Autodesk Inventor part; units mm, degrees
ref_plane "YZ Plane" through (0, 0, 0) normal (1, 0, 0) x (0, 1, 0)
ref_plane "XZ Plane" through (0, 0, 0) normal (0, 1, 0) x (-1, 0, 0)
ref_plane "XY Plane" through (0, 0, 0) normal (0, 0, 1) x (1, 0, 0)
sketch "Sketch1" plane through (0, 0, 0) normal (0, 0, 1) x (1, 0, 0)
  circle A0 centre (45.5, -15.3826) radius 3
  circle A1 centre (-45.5, -15.3826) radius 3
  line L0 (44.6636, 0.7689) -> (35.6636, 0.7689)
  line L1 (33.6636, 2.7689) -> (33.6636, 5.2689)
  line L2 (46.6636, 5.2689) -> (46.6636, 2.7689)
  line L3 (29.9455, -2.1666) -> (-2.0545, -2.1666)
  line L4 (-4.0545, -0.1666) -> (-4.0545, 2.8334)
  line L5 (31.9455, 2.8334) -> (31.9455, -0.1666)
  circle A2 centre (89.024, -15.4039) radius 1.5
  circle A3 centre (65.024, -15.4039) radius 1.5
  circle A4 centre (89.024, 8.5961) radius 1.5
  circle A5 centre (65.024, 8.5961) radius 1.5
  arc A6 (67.8322, 7.6809) -> (67.8322, -14.4886) centre (77.024, -3.4039) ccw
  line L6 (69.3366, 7.4111) -> (71.8641, 3.0334)
  arc A7 (71.8641, 3.0334) -> (71.8641, -9.8411) centre (77.024, -3.4039) ccw
  line L7 (71.8641, -9.8411) -> (69.3366, -14.2188)
  arc A8 (67.8322, -14.4886) -> (69.3366, -14.2188) centre (68.4705, -13.7188) ccw
  arc A9 (69.3366, 7.4111) -> (67.8322, 7.6809) centre (68.4705, 6.9111) ccw
  arc A10 (91.2195, -0.986) -> (72.0202, 10.0988) centre (77.024, -3.4039) ccw
  arc A11 (72.0202, 10.0988) -> (71.5016, 8.6611) centre (72.3677, 9.1611) ccw
  line L8 (74.0291, 4.2834) -> (71.5016, 8.6611)
  arc A12 (85.1787, -2.1539) -> (74.0291, 4.2834) centre (77.024, -3.4039) ccw
  line L9 (90.2337, -2.1539) -> (85.1787, -2.1539)
  arc A13 (90.2337, -2.1539) -> (91.2195, -0.986) centre (90.2337, -1.1539) ccw
  line L10 (85.1787, -4.6539) -> (90.2337, -4.6539)
  arc A14 (91.2195, -5.8218) -> (90.2337, -4.6539) centre (90.2337, -5.6539) ccw
  arc A15 (72.0202, -16.9065) -> (91.2195, -5.8218) centre (77.024, -3.4039) ccw
  arc A16 (71.5016, -15.4688) -> (72.0202, -16.9065) centre (72.3677, -15.9688) ccw
  line L11 (71.5016, -15.4688) -> (74.0291, -11.0911)
  arc A17 (74.0291, -11.0911) -> (85.1787, -4.6539) centre (77.024, -3.4039) ccw
  circle A18 centre (-64.8953, -15.374) radius 1.5
  circle A19 centre (-88.8953, -15.374) radius 1.5
  circle A20 centre (-88.8953, 8.626) radius 1.5
  circle A21 centre (-64.8953, 8.626) radius 1.5
  arc A22 (-62.6997, -0.956) -> (-81.8991, 10.1287) centre (-76.8953, -3.374) ccw
  arc A23 (-81.8991, 10.1287) -> (-82.4176, 8.691) centre (-81.5516, 9.191) ccw
  line L12 (-79.8901, 4.3133) -> (-82.4176, 8.691)
  line L13 (-84.5827, 7.441) -> (-82.0552, 3.0633)
  arc A24 (-84.5827, 7.441) -> (-86.087, 7.7108) centre (-85.4487, 6.941) ccw
  arc A25 (-86.087, 7.7108) -> (-86.087, -14.4587) centre (-76.8953, -3.374) ccw
  arc A26 (-82.0552, 3.0633) -> (-82.0552, -9.8112) centre (-76.8953, -3.374) ccw
  arc A27 (-68.7405, -2.124) -> (-79.8901, 4.3133) centre (-76.8953, -3.374) ccw
  line L14 (-63.6855, -2.124) -> (-68.7405, -2.124)
  arc A28 (-63.6855, -2.124) -> (-62.6997, -0.956) centre (-63.6855, -1.124) ccw
  line L15 (-68.7405, -4.624) -> (-63.6855, -4.624)
  arc A29 (-62.6997, -5.7919) -> (-63.6855, -4.624) centre (-63.6855, -5.624) ccw
  arc A30 (-81.8991, -16.8766) -> (-62.6997, -5.7919) centre (-76.8953, -3.374) ccw
  arc A31 (-79.8901, -11.0612) -> (-68.7405, -4.624) centre (-76.8953, -3.374) ccw
  line L16 (-82.4176, -15.4389) -> (-79.8901, -11.0612)
  arc A32 (-82.4176, -15.4389) -> (-81.8991, -16.8766) centre (-81.5516, -15.9389) ccw
  line L17 (-82.0552, -9.8112) -> (-84.5827, -14.1889)
  arc A33 (-86.087, -14.4587) -> (-84.5827, -14.1889) centre (-85.4487, -13.6889) ccw
  line L18 (-2.0545, 4.8334) -> (29.9455, 4.8334)
  line L19 (35.6636, 7.2689) -> (44.6636, 7.2689)
  arc A34 (-4.0545, -0.1666) -> (-2.0545, -2.1666) centre (-2.0545, -0.1666) ccw
  arc A35 (-2.0545, 4.8334) -> (-4.0545, 2.8334) centre (-2.0545, 2.8334) ccw
  arc A36 (31.9455, 2.8334) -> (29.9455, 4.8334) centre (29.9455, 2.8334) ccw
  arc A37 (29.9455, -2.1666) -> (31.9455, -0.1666) centre (29.9455, -0.1666) ccw
  arc A38 (33.6636, 2.7689) -> (35.6636, 0.7689) centre (35.6636, 2.7689) ccw
  arc A39 (35.6636, 7.2689) -> (33.6636, 5.2689) centre (35.6636, 5.2689) ccw
  arc A40 (46.6636, 5.2689) -> (44.6636, 7.2689) centre (44.6636, 5.2689) ccw
  arc A41 (44.6636, 0.7689) -> (46.6636, 2.7689) centre (44.6636, 2.7689) ccw
  line L20 (-87.4504, 24.6174) -> (-57.4504, 24.6174)
  line L21 (-87.4504, 19.6174) -> (-87.4504, 24.6174)
  line L22 (-87.4504, 19.6174) -> (-57.4504, 19.6174)
  line L23 (-57.4504, 19.6174) -> (-57.4504, 24.6174)
  line L24 (-27.4504, 19.6174) -> (27.5496, 19.6174)
  line L25 (27.5496, 19.6174) -> (27.5496, 24.6174)
  line L26 (-27.4504, 24.6174) -> (27.5496, 24.6174)
  line L27 (-27.4504, 19.6174) -> (-27.4504, 24.6174)
  line L28 (57.5496, 19.6174) -> (87.5496, 19.6174)
  line L29 (87.5496, 19.6174) -> (87.5496, 24.6174)
  line L30 (57.5496, 24.6174) -> (87.5496, 24.6174)
  line L31 (57.5496, 19.6174) -> (57.5496, 24.6174)
  line L32 (-98.9504, -25.3833) -> (-98.9504, -33.3826)
  line L33 (99.0496, -33.3826) -> (-98.9504, -33.3826)
  line L34 (-98.9504, 24.6174) -> (-93.9504, 24.6174)
  line L35 (-93.9504, 24.6174) -> (-93.9504, 9.6159)
  line L36 (-98.9504, 9.6159) -> (-93.9504, 9.6159)
  line L37 (-98.9504, 9.6159) -> (-98.9504, -10.3841)
  line L38 (-98.9504, -10.3841) -> (-93.9504, -10.3841)
  line L39 (-93.9504, -10.3841) -> (-93.9504, -25.3833)
  line L40 (-98.9504, -25.3833) -> (-93.9504, -25.3833)
  line L41 (99.0496, -25.3833) -> (99.0496, -33.3833)
  line L42 (94.0496, -25.3833) -> (99.0496, -25.3833)
  line L43 (94.0496, -10.3841) -> (94.0496, -25.3833)
  line L44 (94.0496, -10.3841) -> (99.0496, -10.3841)
  line L45 (99.0496, 9.6159) -> (99.0496, -10.3841)
  line L46 (94.0496, 9.6159) -> (99.0496, 9.6159)
  line L47 (94.0496, 24.6174) -> (94.0496, 9.6159)
  line L48 (94.0496, 24.6174) -> (99.0496, 24.6174)
  line L49 (-98.9504, 24.6174) -> (-98.9504, 32.6174)
  line L50 (-98.9504, 32.6174) -> (99.0496, 32.6174)
  line L51 (99.0496, 32.6174) -> (99.0496, 24.6174)
  line L52 (-22.6436, -2.2792) -> (-22.6436, -8.2792)
  line L53 (-35.6436, -0.2792) -> (-24.6436, -0.2792)
  line L54 (-24.6436, -10.2792) -> (-35.6436, -10.2792)
  line L55 (-37.6436, -8.2792) -> (-37.6436, -2.2792)
  arc A42 (-35.6436, -0.2792) -> (-37.6436, -2.2792) centre (-35.6436, -2.2792) ccw
  arc A43 (-22.6436, -2.2792) -> (-24.6436, -0.2792) centre (-24.6436, -2.2792) ccw
  arc A44 (-24.6436, -10.2792) -> (-22.6436, -8.2792) centre (-24.6436, -8.2792) ccw
  arc A45 (-37.6436, -8.2792) -> (-35.6436, -10.2792) centre (-35.6436, -8.2792) ccw
  line L56 (-5.5869, 3.8805) -> (-5.5869, -1.877)
  line L57 (-7.5869, -3.877) -> (-13.5192, -3.877)
  line L58 (-15.5192, -1.877) -> (-15.5192, 3.8805)
  line L59 (-13.5192, 5.8805) -> (-7.5869, 5.8805)
  arc A46 (-13.5192, 5.8805) -> (-15.5192, 3.8805) centre (-13.5192, 3.8805) ccw
  arc A47 (-15.5192, -1.877) -> (-13.5192, -3.877) centre (-13.5192, -1.877) ccw
  arc A48 (-5.5869, 3.8805) -> (-7.5869, 5.8805) centre (-7.5869, 3.8805) ccw
  arc A49 (-7.5869, -3.877) -> (-5.5869, -1.877) centre (-7.5869, -1.877) ccw
  point P0 (-90.9348, -30.6649)
  point P1 (27.5, 24.6174)
  point P2 (0, 0)
  point P3 (-22.6436, -0.2792)
  point P4 (-22.6436, -10.2792)
  point P5 (-37.6436, -0.2792)
  point P6 (-37.6436, -10.2792)
  point P7 (-2.0545, 2.8334)
  dimension "d22" = 91
  dimension "d27" = 7
  dimension "d28" = 36
  dimension "d29" = 13
  dimension "d30" = 6.5
  dimension "d35" = 18
  dimension "d36" = 18
  dimension "d37" = 66
  dimension "d38" = 45.5
  dimension "d39" = 6
  dimension "d40" = 6
  dimension "d41" = 198
extrude "Extrusion1" add sketch "Sketch1" along normal blind 5
sketch "Sketch2" plane through (0, 0, 5) normal (0, 0, 1) x (1, 0, 0)
  line L0 (-44.5, 11.026) -> (44.5, 11.026)
  line L1 (48.5, 7.026) -> (48.5, -6.974)
  line L2 (44.5, -10.974) -> (-44.5, -10.974)
  line L3 (-48.5, -6.974) -> (-48.5, 7.026)
  arc A0 (-44.5, 11.026) -> (-48.5, 7.026) centre (-44.5, 7.026) ccw
  arc A1 (48.5, 7.026) -> (44.5, 11.026) centre (44.5, 7.026) ccw
  arc A2 (44.5, -10.974) -> (48.5, -6.974) centre (44.5, -6.974) ccw
  arc A3 (-48.5, -6.974) -> (-44.5, -10.974) centre (-44.5, -6.974) ccw
  line L4 (99.0496, -10.3841) -> (99.0496, 9.6159)
  line L5 (-98.9504, -33.3826) -> (99.0496, -33.3826)
  circle A4 centre (-45.5, -15.3826) radius 3
  circle A5 centre (45.5, -15.3826) radius 3
  arc A6 (-62.6997, -0.956) -> (-81.8991, 10.1287) centre (-76.8953, -3.374) ccw
  point P0 (0, 0)
  point P1 (-76.8953, -3.374)
  dimension "d48" = 4
  dimension "d58" = 97
  dimension "d59" = 22
  dimension "d60" = 50.5496
  dimension "d61" = 22.4087
extrude "Extrusion2" cut sketch "Sketch2" against normal up to next contours L0 A1 L1 A2 L2 A3 L3 A0
sketch "Sketch3" plane through (0, 0, 5) normal (0, 0, 1) x (1, 0, 0)
  line L0 (-92.421, 12.1859) -> (-62.2986, 12.1859)
  line L1 (-62.2986, 12.1859) -> (-62.2986, -19.0319)
  line L2 (-62.2986, -19.0319) -> (-92.421, -19.0319)
  line L3 (-92.421, -19.0319) -> (-92.421, 12.1859)
  line L4 (-92.421, 12.1859) -> (-62.2986, -19.0319) construction
  line L5 (-62.2986, 12.1859) -> (-92.421, -19.0319) construction
  line L6 (62.2986, 11.0377) -> (92.6949, 11.0377)
  line L7 (92.6949, 11.0377) -> (92.6949, -17.8837)
  line L8 (92.6949, -17.8837) -> (62.2986, -17.8837)
  line L9 (62.2986, -17.8837) -> (62.2986, 11.0377)
  line L10 (62.2986, 11.0377) -> (92.6949, -17.8837) construction
  line L11 (92.6949, 11.0377) -> (62.2986, -17.8837) construction
  point P0 (0, 0)
  point P1 (-77.3598, -3.423)
  point P2 (77.4968, -3.423)
extrude "Extrusion3" add sketch "Sketch3" against normal blind 5
sketch "Sketch4" plane through (0, 0, 5) normal (0, 0, 1) x (1, 0, 0)
  arc A0 (44.5, -10.974) -> (48.5, -6.974) centre (44.5, -6.974) ccw
  line L0 (44.5, -10.974) -> (-44.5, -10.974)
  arc A1 (-48.5, -6.974) -> (-44.5, -10.974) centre (-44.5, -6.974) ccw
  line L1 (-48.5, -6.974) -> (-48.5, 7.026)
  arc A2 (-44.5, 11.026) -> (-48.5, 7.026) centre (-44.5, 7.026) ccw
  line L2 (-44.5, 11.026) -> (44.5, 11.026)
  arc A3 (48.5, 7.026) -> (44.5, 11.026) centre (44.5, 7.026) ccw
  line L3 (48.5, 7.026) -> (48.5, -6.974)
  line L4 (-98.9504, -33.3826) -> (99.0496, -33.3826)
  line L5 (99.0496, -33.3826) -> (99.0496, -25.3833)
  line L6 (99.0496, -25.3833) -> (94.0496, -25.3833)
  line L7 (94.0496, -25.3833) -> (94.0496, -10.3841)
  line L8 (94.0496, -10.3841) -> (99.0496, -10.3841)
  line L9 (99.0496, -10.3841) -> (99.0496, 9.6159)
  line L10 (99.0496, 9.6159) -> (94.0496, 9.6159)
  line L11 (94.0496, 9.6159) -> (94.0496, 24.6174)
  line L12 (94.0496, 24.6174) -> (99.0496, 24.6174)
  line L13 (99.0496, 24.6174) -> (99.0496, 32.6174)
  line L14 (99.0496, 32.6174) -> (-98.9504, 32.6174)
  line L15 (-98.9504, 32.6174) -> (-98.9504, 24.6174)
  line L16 (-98.9504, 24.6174) -> (-93.9504, 24.6174)
  line L17 (-93.9504, 24.6174) -> (-93.9504, 9.6159)
  line L18 (-93.9504, 9.6159) -> (-98.9504, 9.6159)
  line L19 (-98.9504, 9.6159) -> (-98.9504, -10.3841)
  line L20 (-98.9504, -10.3841) -> (-93.9504, -10.3841)
  line L21 (-93.9504, -10.3841) -> (-93.9504, -25.3833)
  line L22 (-93.9504, -25.3833) -> (-98.9504, -25.3833)
  line L23 (-98.9504, -25.3833) -> (-98.9504, -33.3826)
  circle A4 centre (45.5, -15.3826) radius 3
  circle A5 centre (-45.5, -15.3826) radius 3
  line L24 (57.5496, 24.6174) -> (87.5496, 24.6174)
  line L25 (87.5496, 24.6174) -> (87.5496, 19.6174)
  line L26 (87.5496, 19.6174) -> (57.5496, 19.6174)
  line L27 (57.5496, 19.6174) -> (57.5496, 24.6174)
  line L28 (-27.4504, 24.6174) -> (27.5496, 24.6174)
  line L29 (27.5496, 24.6174) -> (27.5496, 19.6174)
  line L30 (27.5496, 19.6174) -> (-27.4504, 19.6174)
  line L31 (-27.4504, 19.6174) -> (-27.4504, 24.6174)
  line L32 (-87.4504, 19.6174) -> (-87.4504, 24.6174)
  line L33 (-87.4504, 24.6174) -> (-57.4504, 24.6174)
  line L34 (-57.4504, 24.6174) -> (-57.4504, 19.6174)
  line L35 (-57.4504, 19.6174) -> (-87.4504, 19.6174)
  point P0 (0, 0)
properties part number "case bottom back" material "Titanium"
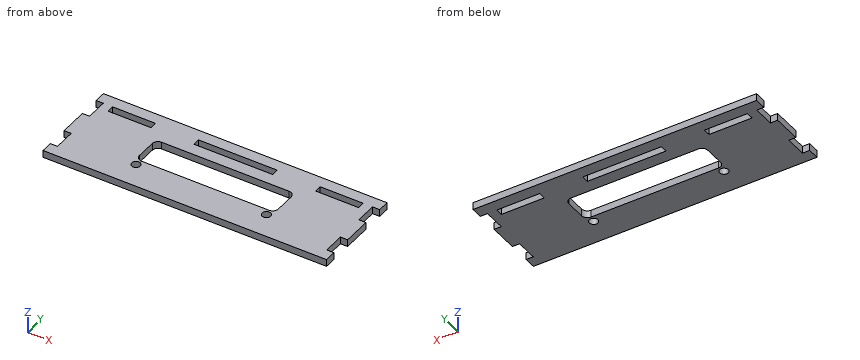
For this review, take the finished solid that the model builds, in its own axes (mm). Give positions to 0.01 mm unless a question says otherwise; leave off trailing zeros. Order: outer loops, then holes, each group sorted by start corner. A loop starts at its lowest first (then second) coordinate and runs counter-clockwise, first axis right, second up. Notation, with made-up numbers: (12, -16) - (60, -16) arc R5 ccw to (60, -12) - close; hole circle Ø6 at (77.5, -28). An arc over 180 degrees is marked (long way). Answer as a JSON object with one key per item and string values. Group by question number.
Item 1: Take a section at A-A on x = -68. Give the boundary of the cut face in (y, z), and give its area (3 significant figures).
Item 2: Take a section at B-B on y = -21.5. Give the boundary of the cut face in (x, z), and give its area (3 significant figures).
Item 3: Wall thickness on line 1 along X through (y, z) = (20, 1.3); line 2 along X through (y, z) = (-7.5, 2.45); line 3 along Y through (x, z) = (-0.5, 4.35): over which ranges is each line inside the solid? List them lowest first.
Item 4: Clearance check with flat-ended pins moving along their axes: pin 1 Ø2.5 at (y, z) = (22.5, 2) entering from +X; pin 2 Ø2.5 at (y, z) = (-16.5, 2) entering from -X; pin 3 Ø5 at (x, y) = (45.5, -15.38) entering from +Z. State where each tip first meets the part, or that it passes through.
Item 5: Take a section at C-C on z = 3.75. Give the number of separate pieces and of enclosed holes in the cut face, and give its area (3 significant figures).
Reported:
{
 "1": {"outline": "(-33.38, 0) - (19.62, 0) - (19.62, 5) - (-33.38, 5) - close; (24.62, 0) - (32.62, 0) - (32.62, 5) - (24.62, 5) - close", "area": "305 mm^2"},
 "2": {"outline": "(-93.95, 0) - (94.05, 0) - (94.05, 5) - (-93.95, 5) - close", "area": "940 mm^2"},
 "3": {"line 1": "-93.95 to -87.45, -57.45 to -27.45, 27.55 to 57.55, 87.55 to 94.05", "line 2": "-98.95 to -48.47, 48.47 to 99.05", "line 3": "-33.38 to -10.97, 11.03 to 19.62, 24.62 to 32.62"},
 "4": {"pin 1": "x = 94.05", "pin 2": "x = -93.95", "pin 3": "through"},
 "5": {"separate pieces": "1", "enclosed holes": "6", "area": "10,000 mm^2"}
}
